Part model, mm, in its own coordinate system. A direction names the side the tool comes from. Coordinates: 2 decimals unless noted, no trailing zeros. Loops run counter-clockwise (first coordinate to the right, second up) from the corner with the lowest first, then second, coordinate; pieces in that order, holes last. Notation, with made-up numbers: M 53,43 L 105,43 A17 cw 105,52 Z; hole C 42.5,23 d11. An arc over 180 degrees is marked long. Answer as a JSON object with one key per item and string values. Group by question number.
1. 3-axis set-ups, long thin cutter, end or side, ignore diameter. For faces 5 (the face through (-10, -20, -26)), 6 (the face through (-19.1, -19.72, 0.27)), 7 (the face through (-6, -5, -33)): which of +Z, -Z, +X, -X, +Y, -Y reach the whole face in a straight line?
2. Drill centre lines: L1, parallel to Z at x = -6.5, y = -22.5; L2, parallel to Z at x = -5.75, y = -30; L3, parallel to X at y = -13, z = 22. Where is each one in solid material? Low to high.
3. Saw through at B-B on x = -4.75. Write the cut outline in (y, z), then the cut area to 3 significant figures.
4. Drop flat-ended pins along their axis: pin 1 Ø6 at (y, z) = (-18.5, 20) entering from -X; pin 2 Ø5 at (y, z) = (-20, 10) entering from +X; pin 3 Ø2 at (x, y) = (-15, -34) entering from -Z. Give the stop position or say it passes through.
5. Saw through at A-A on z = -36.5. Write the cut outline in (x, y), then the cut area to 3 significant figures.
6. Saw through at C-C on y = -11. Write the cut outline in (x, z), then the cut area to 3 significant figures.
7. Saw through at D-D on x = -14.5. Write the cut outline in (y, z).
8. Mould opens along Z. For faces 1 (the face through (-10, -20, 22)), 2 (the face through (-6, -20, -28)), 3 (the face through (-6, -20, -43)), 4 (the face through (-6, -34.421, -33)) say: released by +Z, released by -Z, zero draft, split by the parting line, or undercut.
from build123d import *

# Parameters (mm, degrees)
F1_DEPTH = 40
F2_W     = 29.421238
F2_H     = 10
F3_DEPTH = 8.001


with BuildPart() as f1:
    # F0 (on Front) → F1 (new body)
    with BuildSketch(Plane.XZ):
        with BuildLine():
            ThreePointArc((-2, -15.975293), (-16.1, 0), (-2, 15.975293))
            Line((-2, 15.975293), (-2, 28))
            Line((-2, 28), (-10, 28))
            Line((-10, 28), (-10, 16.272984))
            ThreePointArc((-10, 16.272984), (-19.1, 0), (-10, -16.272984))
            Line((-10, -16.272984), (-10, -28))
            Line((-10, -28), (-10, -43))
            Line((-10, -43), (-2, -43))
            Line((-2, -43), (-2, -28))
            Line((-2, -28), (-2, -15.975293))
        make_face()
    extrude(amount=F1_DEPTH)

    # F2 (on face) → F3 (cut, through all)
    with BuildSketch(Plane(origin=(-10, 0, 0), x_dir=(0, -1, 0), z_dir=(-1, 0, 0))):
        with Locations((19.710619, -33)):
            Rectangle(F2_W, F2_H)
    extrude(amount=-F3_DEPTH, mode=Mode.SUBTRACT)


solid = f1.part
Outcome:
{
 "1": {"face 5": "-Z, -X, +Y, -Y", "face 6": "-X, +Y, -Y", "face 7": "+X, -X"},
 "2": {"L1": "z = -43 to -38, -28 to -14.73, 14.73 to 28", "L2": "z = -43 to -38, -28 to -15.04, 15.04 to 28", "L3": "x = -10 to -2"},
 "3": {"outline": "M -40,-43 L 0,-43 L 0,-15.38 L -40,-15.38 Z; M -40,15.38 L 0,15.38 L 0,28 L -40,28 Z; hole M -34.42,-38 L -5,-38 L -5,-28 L -34.42,-28 Z", "area": "1,320 mm²"},
 "4": {"pin 1": "stops at x = -10", "pin 2": "stops at x = -10.15", "pin 3": "stops at z = -12.99"},
 "5": {"outline": "M -10,-40 L -2,-40 L -2,-34.42 L -10,-34.42 Z; M -10,-5 L -2,-5 L -2,0 L -10,0 Z", "area": "84.6 mm²"},
 "6": {"outline": "M -10,-43 L -2,-43 L -2,-38 L -10,-38 Z; M -10,-28 L -2,-28 L -2,-15.98 A16.1 cw -2,15.98 L -2,28 L -10,28 L -10,16.27 A19.1 ccw -10,-16.27 Z", "area": "354 mm²"},
 "7": {"outline": "M -40,-12.43 L 0,-12.43 L 0,-7 L -40,-7 Z; M -40,7 L 0,7 L 0,12.43 L -40,12.43 Z"},
 "8": {"face 1": "zero draft", "face 2": "undercut", "face 3": "released by -Z", "face 4": "undercut"}
}
